Part model, mm, in its own coordinate system. Face numbers are marked on the shaded views. A direction names the side the tool comes from. Coordinates: 2 decimals unless noted, no trailing zeros. Order: outer loops, then holes, each group sorted by start corner. A loop starts at its lowest first (then second) coordinate and runs counter-clockwise, first axis right, second up.
1) Cut at B-B (x = -64). List the corners of the cut face in (y, z).
2) Wall check: L1, parallel to Y at x = -188.5, z = -206; L2, parallel to X at y = 8.5, z = -275; L3, parallel to Y at x = -52.5, z = -169.5. Give the ranges that are in metal, low to high.
3) Cut at A-A (z = -281). List the corners of the cut face in (x, y).
4) Pin check, flat tips, straight feed: pin 1 Ø8 at (x, z) = (-59.5, -228) entering from -Y; pin 2 Ø10 at (x, z) = (-69.5, -295) entering from +Y; pin 3 Ø8 at (y, z) = (104.5, -256.5) entering from +X; pin 4 Ø6 at (y, z) = (76, -234.5) entering from -X. Stop position of each tip, or through.
5) Tool access for the marked faces 1, 2, 3 and 4: list every direction of +Z, -Z, +X, -X, +Y, -Y with a clear straight run to the whole face (end or side of a thin tool).
6) Cut at C-C (y = 118.5). List the corners of the cut face in (x, z).
7) Cut at D-D (z = -184.5). List the corners of the cut face in (x, y), and give its area (3 significant figures).
8) Mould opens along Y. For the marked faces 5, 6 and 7 say: +Y half, -Y half, draft (parallel to the pull), parting line (faces both ways), or undercut.
Autodesk Inventor part; units mm, degrees
ref_plane "YZ Plane" through (0, 0, 0) normal (1, 0, 0) x (0, 1, 0)
ref_plane "XZ Plane" through (0, 0, 0) normal (0, 1, 0) x (-1, 0, 0)
ref_plane "XY Plane" through (0, 0, 0) normal (0, 0, 1) x (1, 0, 0)
sketch "Sketch1" plane through (0, 0, 0) normal (0, 1, 0) x (-1, 0, 0)
  circle A0 centre (0, 0) radius 145
  circle A1 centre (0, 0) radius 325
  line L0 (0, 0) -> (325, 0)
  line L1 (0, 0) -> (0, -325)
  line L2 (0, 0) -> (229.8097, -229.8097)
  line L3 (229.8097, -229.8097) -> (0, -145) construction
  line L4 (1.3869, -199.3328) -> (139.9689, -141.9303)
  line L5 (139.9689, -141.9303) -> (178.2372, -234.3183)
  line L6 (178.2372, -234.3183) -> (39.6553, -291.7208)
  line L7 (39.6553, -291.7208) -> (1.3869, -199.3328)
  line L8 (102.5305, -102.5305) -> (0, -325) construction
  circle A2 centre (0, 0) radius 306.4883 construction
  line L9 (178.2372, -234.3183) -> (1.3869, -199.3328) construction
  line L10 (139.9689, -141.9303) -> (39.6553, -291.7208) construction
  line L11 (89.8121, -216.8255) -> (108.9463, -263.0195) construction
  line L12 (0, 0) -> (124.3721, -300.2608) construction
  line L13 (199.3328, -1.3869) -> (291.7208, -39.6553)
  line L14 (141.9303, -139.9689) -> (199.3328, -1.3869)
  line L15 (234.3183, -178.2372) -> (141.9303, -139.9689)
  line L16 (291.7208, -39.6553) -> (234.3183, -178.2372)
  line L17 (141.9303, 139.9689) -> (234.3183, 178.2372)
  line L18 (199.3328, 1.3869) -> (141.9303, 139.9689)
  line L19 (291.7208, 39.6553) -> (199.3328, 1.3869)
  line L20 (234.3183, 178.2372) -> (291.7208, 39.6553)
  line L21 (1.3869, 199.3328) -> (39.6553, 291.7208)
  line L22 (139.9689, 141.9303) -> (1.3869, 199.3328)
  line L23 (178.2372, 234.3183) -> (139.9689, 141.9303)
  line L24 (39.6553, 291.7208) -> (178.2372, 234.3183)
  line L25 (-139.9689, 141.9303) -> (-178.2372, 234.3183)
  line L26 (-1.3869, 199.3328) -> (-139.9689, 141.9303)
  line L27 (-39.6553, 291.7208) -> (-1.3869, 199.3328)
  line L28 (-178.2372, 234.3183) -> (-39.6553, 291.7208)
  line L29 (-199.3328, 1.3869) -> (-291.7208, 39.6553)
  line L30 (-141.9303, 139.9689) -> (-199.3328, 1.3869)
  line L31 (-234.3183, 178.2372) -> (-141.9303, 139.9689)
  line L32 (-291.7208, 39.6553) -> (-234.3183, 178.2372)
  line L33 (-141.9303, -139.9689) -> (-234.3183, -178.2372)
  line L34 (-199.3328, -1.3869) -> (-141.9303, -139.9689)
  line L35 (-291.7208, -39.6553) -> (-199.3328, -1.3869)
  line L36 (-234.3183, -178.2372) -> (-291.7208, -39.6553)
  line L37 (-1.3869, -199.3328) -> (-39.6553, -291.7208)
  line L38 (-139.9689, -141.9303) -> (-1.3869, -199.3328)
  line L39 (-178.2372, -234.3183) -> (-139.9689, -141.9303)
  line L40 (-39.6553, -291.7208) -> (-178.2372, -234.3183)
  circle A3 centre (0, 0) radius 235 construction
  point P0 (263.0195, -108.9463)
  point P1 (263.0195, 108.9463)
  point P2 (108.9463, 263.0195)
  point P3 (-108.9463, 263.0195)
  point P4 (-263.0195, 108.9463)
  point P5 (-263.0195, -108.9463)
  point P6 (-108.9463, -263.0195)
  dimension "d1" = 180
  dimension "d3" = 45
  dimension "d4" = 650
  dimension "d11" = 150
  dimension "d12" = 100
  dimension "d13" = 22.5
  dimension "d16" = 360
  dimension "d18" = 90
extrude "Extrusion1" add sketch "Sketch1" along normal blind 10 contours A0 L2 A1 L1 | L4 L5 L6 L7
sketch "Sketch2" plane through (0, 10, 0) normal (0, 1, 0) x (1, 0, 0)
  circle A0 centre (0, 0) radius 325
  circle A1 centre (0, 0) radius 145
  line L0 (0, 0) -> (-325, 0)
  line L1 (0, 145) -> (0, 325)
  line L2 (0, 0) -> (0, 325)
  arc A2 (0, 325) -> (-229.8097, 229.8097) centre (0, 0) ccw
  line L3 (0, 0) -> (-229.8097, 229.8097)
  circle A3 centre (0, 0) radius 235 construction
  line L4 (0, 0) -> (-124.3721, 300.2608) construction
  line L5 (-1.5055, 199.619) -> (-140.0874, 142.2165)
  line L6 (-140.0874, 142.2165) -> (-178.3557, 234.6044)
  line L7 (-178.3557, 234.6044) -> (-39.7738, 292.0069)
  line L8 (-39.7738, 292.0069) -> (-1.5055, 199.619)
  line L9 (-1.5055, 199.619) -> (-178.3557, 234.6044) construction
  line L10 (-140.0874, 142.2165) -> (-39.7738, 292.0069) construction
  circle A4 centre (0, 0) radius 185
  line L11 (-199.619, 1.5055) -> (-292.0069, 39.7738)
  line L12 (-142.2165, 140.0874) -> (-199.619, 1.5055)
  line L13 (-234.6044, 178.3557) -> (-142.2165, 140.0874)
  line L14 (-292.0069, 39.7738) -> (-234.6044, 178.3557)
  line L15 (-199.619, 1.5055) -> (-234.6044, 178.3557) construction
  line L16 (-142.2165, 140.0874) -> (-292.0069, 39.7738) construction
  line L17 (-142.2165, -140.0874) -> (-234.6044, -178.3557)
  line L18 (-199.619, -1.5055) -> (-142.2165, -140.0874)
  line L19 (-292.0069, -39.7738) -> (-199.619, -1.5055)
  line L20 (-234.6044, -178.3557) -> (-292.0069, -39.7738)
  line L21 (-142.2165, -140.0874) -> (-292.0069, -39.7738) construction
  line L22 (-199.619, -1.5055) -> (-234.6044, -178.3557) construction
  line L23 (-1.5055, -199.619) -> (-39.7738, -292.0069)
  line L24 (-140.0874, -142.2165) -> (-1.5055, -199.619)
  line L25 (-178.3557, -234.6044) -> (-140.0874, -142.2165)
  line L26 (-39.7738, -292.0069) -> (-178.3557, -234.6044)
  line L27 (-1.5055, -199.619) -> (-178.3557, -234.6044) construction
  line L28 (-140.0874, -142.2165) -> (-39.7738, -292.0069) construction
  line L29 (140.0874, -142.2165) -> (178.3557, -234.6044)
  line L30 (1.5055, -199.619) -> (140.0874, -142.2165)
  line L31 (39.7738, -292.0069) -> (1.5055, -199.619)
  line L32 (178.3557, -234.6044) -> (39.7738, -292.0069)
  line L33 (140.0874, -142.2165) -> (39.7738, -292.0069) construction
  line L34 (1.5055, -199.619) -> (178.3557, -234.6044) construction
  line L35 (199.619, -1.5055) -> (292.0069, -39.7738)
  line L36 (142.2165, -140.0874) -> (199.619, -1.5055)
  line L37 (234.6044, -178.3557) -> (142.2165, -140.0874)
  line L38 (292.0069, -39.7738) -> (234.6044, -178.3557)
  line L39 (199.619, -1.5055) -> (234.6044, -178.3557) construction
  line L40 (142.2165, -140.0874) -> (292.0069, -39.7738) construction
  line L41 (142.2165, 140.0874) -> (234.6044, 178.3557)
  line L42 (199.619, 1.5055) -> (142.2165, 140.0874)
  line L43 (292.0069, 39.7738) -> (199.619, 1.5055)
  line L44 (234.6044, 178.3557) -> (292.0069, 39.7738)
  line L45 (142.2165, 140.0874) -> (292.0069, 39.7738) construction
  line L46 (199.619, 1.5055) -> (234.6044, 178.3557) construction
  line L47 (1.5055, 199.619) -> (39.7738, 292.0069)
  line L48 (140.0874, 142.2165) -> (1.5055, 199.619)
  line L49 (178.3557, 234.6044) -> (140.0874, 142.2165)
  line L50 (39.7738, 292.0069) -> (178.3557, 234.6044)
  line L51 (1.5055, 199.619) -> (178.3557, 234.6044) construction
  line L52 (140.0874, 142.2165) -> (39.7738, 292.0069) construction
  line L53 (-151.5679, 169.9328) -> (-156.5679, 167.8618)
  line L54 (-156.5679, 167.8618) -> (-173.1364, 207.8618)
  line L55 (-173.1364, 207.8618) -> (-168.1364, 209.9328)
  line L56 (-168.1364, 209.9328) -> (-151.5679, 169.9328)
  line L57 (-151.5679, 169.9328) -> (-173.1364, 207.8618) construction
  line L58 (-156.5679, 167.8618) -> (-168.1364, 209.9328) construction
  line L59 (-12.986, 227.3354) -> (-7.986, 229.4064)
  line L60 (-7.986, 229.4064) -> (-24.5545, 269.4064)
  line L61 (-24.5545, 269.4064) -> (-29.5545, 267.3354)
  line L62 (-12.986, 227.3354) -> (-24.5545, 269.4064) construction
  line L63 (-7.986, 229.4064) -> (-29.5545, 267.3354) construction
  line L64 (-111.6098, 154.0123) -> (-121.6098, 149.8701)
  line L65 (-121.6098, 149.8701) -> (-117.8819, 140.8701)
  line L66 (-117.8819, 140.8701) -> (-107.8819, 145.0123)
  line L67 (-107.8819, 145.0123) -> (-111.6098, 154.0123)
  line L68 (-111.6098, 154.0123) -> (-117.8819, 140.8701) construction
  line L69 (-121.6098, 149.8701) -> (-107.8819, 145.0123) construction
  point P0 (-89.9306, 217.1117)
  point P1 (-217.1117, 89.9306)
  point P2 (-217.1117, -89.9306)
  point P3 (-89.9306, -217.1117)
  point P4 (89.9306, -217.1117)
  point P5 (217.1117, -89.9306)
  point P6 (217.1117, 89.9306)
  point P7 (89.9306, 217.1117)
  point P8 (-68.8241, 166.1562)
  point P9 (-29.5545, 267.3354)
  point P10 (-12.986, 227.3354)
  point P11 (-151.5679, 169.9328)
  dimension "d22" = 180
  dimension "d23" = 650
  dimension "d24" = 90
  dimension "d25" = 100
  dimension "d26" = 150
  dimension "d27" = 40
  dimension "d30" = 360
  dimension "d32" = 40
  dimension "d33" = 5
  dimension "d34" = 9
  dimension "d35" = 10
  dimension "d39" = 30
  dimension "d40" = 20
extrude "Extrusion2" add sketch "Sketch2" along normal blind 140 contours L65 L5 L67 A4 | A4 L67 L66 L65 | L8 L61 L60 L59 | L53 L54 L55 L6
ref_plane "Work Plane1" through (0, 80, 0) normal (0, 1, 0) x (1, 0, 0)
sketch "Sketch4" plane through (0, 80, 0) normal (0, 1, 0) x (1, 0, 0)
  line L0 (-24.5545, 269.4064) -> (-7.986, 229.4064)
  line L1 (-7.986, 229.4064) -> (-12.986, 227.3354)
  line L2 (-12.986, 227.3354) -> (-29.5545, 267.3354)
  line L3 (-29.5545, 267.3354) -> (-24.5545, 269.4064)
  line L4 (-156.5679, 167.8618) -> (-173.1364, 207.8618)
  line L5 (-173.1364, 207.8618) -> (-168.1364, 209.9328)
  line L6 (-168.1364, 209.9328) -> (-151.5679, 169.9328)
  line L7 (-151.5679, 169.9328) -> (-156.5679, 167.8618)
  line L8 (-107.8819, 145.0123) -> (-117.8819, 140.8701)
  line L9 (-117.8819, 140.8701) -> (-121.6098, 149.8701)
  line L10 (-121.6098, 149.8701) -> (-111.6098, 154.0123)
  line L11 (-111.6098, 154.0123) -> (-107.8819, 145.0123)
  arc A0 (0, 145) -> (-102.5305, 102.5305) centre (0, 0) ccw
  line L12 (0, 145) -> (0, 325)
  arc A1 (0, 325) -> (-229.8097, 229.8097) centre (0, 0) ccw
  line L13 (-229.8097, 229.8097) -> (-102.5305, 102.5305)
  arc A2 (0, 180) -> (-127.2792, 127.2792) centre (0, 0) ccw
  dimension "d44" = 35
extrude "Extrusion3" add sketch "Sketch4" along normal blind 10 contours A2 L13 A1 L12
properties part number "Carousel Container Plate"
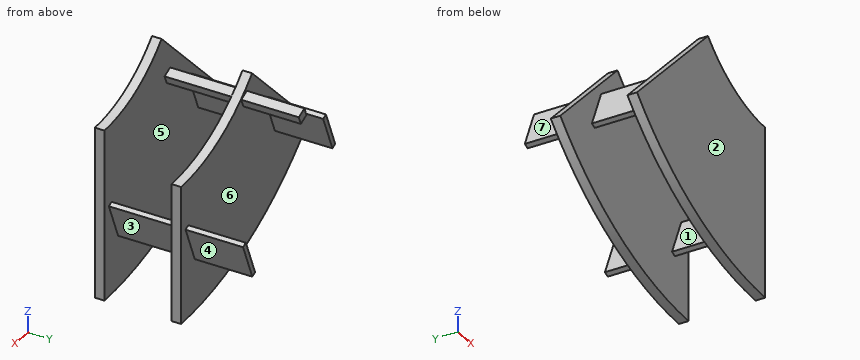
Geometry check:
1. outline: (0, -318.64) - (10, -318.64) - (10, -130.11) - (0, -130.11) - close; (80, -318.64) - (90, -318.64) - (90, -168.24) - (80, -168.24) - close
2. L1: y = 0 to 10, 80 to 90
2. L2: x = -173.21 to 0
2. L3: y = 0 to 10
3. outline: (-163.29, 0) - (0, 0) - (0, 10) - (-163.29, 10) - close; (-163.29, 80) - (0, 80) - (0, 90) - (-163.29, 90) - close
4. pin 1: stops at y = 0
4. pin 2: stops at y = 90
4. pin 3: stops at x = -17.55
4. pin 4: stops at x = -17.2
5. face 1: +Z, -X
5. face 2: +Z, -Z, +X, -X, -Y
5. face 3: -Z, +X
5. face 4: -Z, +X, +Y
6. outline: (-173.14, -207.86) - (-168.14, -209.93) - (-151.57, -169.93) - (-156.57, -167.86) - close; (-121.61, -149.87) - (-111.61, -154.01) - (-107.88, -145.01) - (-117.88, -140.87) - close; (-29.55, -267.34) - (-24.55, -269.41) - (-7.99, -229.41) - (-12.99, -227.34) - close
7. outline: (-184.5, 0) - (0, 0) - (0, 10) - (-157.6, 10) - (-157.6, 80) - (0, 80) - (0, 90) - (-157.6, 90) - (-157.6, 150) - (-163.46, 150) - (-163.46, 90) - (-184.5, 90) - (-184.5, 80) - (-163.46, 80) - (-163.46, 10) - (-184.5, 10) - close
7. area: 4,450 mm2
8. face 5: undercut
8. face 6: +Y half
8. face 7: draft
